Could you check a few things on this drawing? It's one solid part, dimensions in mm from its lowest x, y, z. A direction names the side the tool comes from. Give positions to 0.01 mm unless a question says otherwise; leave off trailing zeros. Loops run counter-clockwise (first coordinate to the right, second up) from the corner with the lowest first, then second, coordinate; pieces in that order, holes last. Notation, with made-up numbers: (54.5, 23) - (89.5, 23) arc R35 ccw to (89.5, 57) - close; hole circle Ø11 at (32.25, 57.25). An arc over 180 degrees is marked (long way). Use CSV: the item, a comma, the result in double quotes.
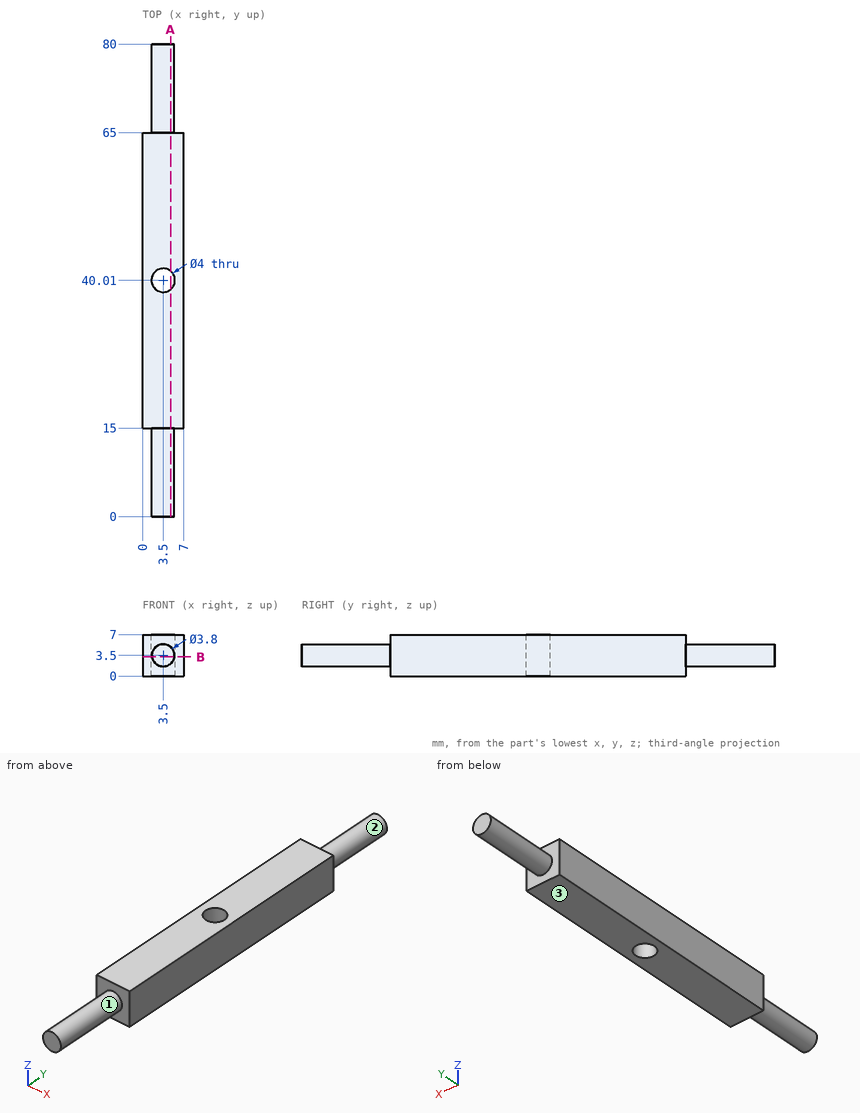
1) I need wall thicknesses on line 1 along Y through (x, z) = (3.5, 5); line 2 along Y through (x, z) = (3.75, 1) (1 decimal); line 3 along Y through (x, z) = (6.75, 1). Which ranges of each line are inside material? Lowest first, please.
Answer below:
line 1,"y = 0 to 38.01, 42.01 to 80"
line 2,"y = 15 to 38, 42 to 65"
line 3,"y = 15 to 65"
2) Suppose I cut it at B-B (z = 3.25). Please give me the cut outline in (x, y).
Answer below:
outline,"(0, 15) - (1.62, 15) - (1.62, 0) - (5.38, 0) - (5.38, 15) - (7, 15) - (7, 65) - (5.38, 65) - (5.38, 80) - (1.62, 80) - (1.62, 65) - (0, 65) - close; hole circle Ø4 at (3.5, 40.01)"
3) Suppose I cut it at A-A (x = 4.75). Please give me the cut outline in (y, z), plus the area to 3 significant figures.
Answer below:
outline,"(0, 2.07) - (15, 2.07) - (15, 0) - (38.45, 0) - (38.45, 7) - (15, 7) - (15, 4.93) - (0, 4.93) - close; (41.57, 0) - (65, 0) - (65, 2.07) - (80, 2.07) - (80, 4.93) - (65, 4.93) - (65, 7) - (41.57, 7) - close"
area,"414 mm2"
4) Which directions (+Z, -Z, +X, -X, +Y, -Y) give clear straight access to the entire face, cutting with the end or side of a thin tool? Please do the marked faces 1, 2 and 3.
Answer below:
face 1,"-Y"
face 2,"+Y"
face 3,"-Z, +X, -X, +Y, -Y"
5) I'm going to push a flat-ended pin straight in: P1, Ø1.5, axis at x = 1.5, y = 71.5, coming from the -Z side. Where does the tip first touch, or does it pass through?
Answer below:
P1,"stops at z = 2.07"
